from build123d import *

# Parameters (mm, degrees)
SKETCH008_W       = 45.6
SKETCH008_H       = 150
PAD004_DEPTH      = 42
PAD004_DEPTH_BACK = 10
SKETCH009_R       = 4
POCKET003_DEPTH   = 52.001
POCKET004_DEPTH   = 7
POCKET005_DEPTH   = 7
SKETCH011_R       = 4
POCKET007_DEPTH   = 45.601


with BuildPart() as part:
    # Sketch008 → Pad004 (new body, two sides)
    with BuildSketch(Plane(origin=(0, 0, 0), x_dir=(-1, 0, 0), z_dir=(0, 1, 0))) as pad004_sk:
        with Locations((214, 75)):
            Rectangle(SKETCH008_W, SKETCH008_H)
    extrude(amount=PAD004_DEPTH)
    extrude(pad004_sk.sketch, amount=-PAD004_DEPTH_BACK)

    # Sketch009 (on Face6 of Pad004) → Pocket003 (cut, through all)
    with BuildSketch(Plane(origin=(0, 42, 0), x_dir=(1, 0, 0), z_dir=(0, 1, 0))):
        with Locations((-211.172606, -26)):
            Circle(SKETCH009_R)
        with Locations((-211.172606, -124)):
            Circle(SKETCH009_R)
    extrude(amount=-POCKET003_DEPTH, mode=Mode.SUBTRACT)

    # Sketch010 (on Face4 of Pocket003) → Pocket004 (cut)
    with BuildSketch(Plane.XZ.offset(10)):
        Polygon((-207.672606, 117.937822), (-204.172606, 124), (-207.672606, 130.062178), (-214.672606, 130.062178), (-218.172606, 124), (-214.672606, 117.937822), align=None)
        Polygon((-207.672606, 19.937822), (-204.172606, 26), (-207.672606, 32.062178), (-214.672606, 32.062178), (-218.172606, 26), (-214.672606, 19.937822), align=None)
    extrude(amount=-POCKET004_DEPTH, mode=Mode.SUBTRACT)

    # Sketch010 (on Face4 of Pocket003) → Pocket005 (cut)
    with BuildSketch(Plane.XZ.offset(10)):
        Polygon((-207.672606, 117.937822), (-204.172606, 124), (-207.672606, 130.062178), (-214.672606, 130.062178), (-218.172606, 124), (-214.672606, 117.937822), align=None)
        Polygon((-207.672606, 19.937822), (-204.172606, 26), (-207.672606, 32.062178), (-214.672606, 32.062178), (-218.172606, 26), (-214.672606, 19.937822), align=None)
    extrude(amount=-POCKET005_DEPTH, mode=Mode.SUBTRACT)

    # Sketch011 → Pocket007 (cut, through all)
    with BuildSketch(Plane(origin=(-191.2, 0, 0), x_dir=(0, -1, 0), z_dir=(-1, 0, 0))):
        with Locations((-16, 135)):
            Circle(SKETCH011_R)
        with Locations((-16, 75)):
            Circle(SKETCH011_R)
        with Locations((-16, 15)):
            Circle(SKETCH011_R)
    extrude(amount=POCKET007_DEPTH, mode=Mode.SUBTRACT)


solid = part.part
The listing builds one solid part. Answer for the finished solid, in the listing's coordinates (mm). A direction names the side the tool comes from. Round coordinates to 2 decimals unless told otherwise and drop trailing zeros. Loops run counter-clockwise (first coordinate to the right, second up) from the corner with the lowest first, then second, coordinate; pieces in that order, holes last. Notation, with made-up numbers: M -10.5,-19.75 L -0.5,-19.75 A27 cw -0.5,19.25 Z; hole C 34,2.5 d4. An arc over 180 degrees is marked long. Write each question's results on one line, items separated by ' | '. Start each with the question number.
1) Find section B-B on y = -5. Write down the section's boundary in (x, z), plus the area to 3 significant figures.
2) Straight lines are drawn through the part: probe 1 along Y at (x, z) = (-215, 135); probe 2 along X at (y, z) = (20.5, 124); probe 3 along Z at (x, y) = (-222.5, 16). For each, find the intervals that lie inside material, in ascending order.
3) Which of the six approach directions +Z, -Z, +X, -X, +Y, -Y give full straight-line access (tool end or side, diameter ignored) to faces 1 (the flat face through (-216.447, -6.549, 121.011)), 2 (the cylindrical face through (-213.68, 18.95, 17.7))?
4) Find section A-A on z = 75. Write down the section's boundary in (x, y).
5) This flat-tipped pin is pushed along its axis until it touches: pin 1 (5 mm diameter, centred on x = -211.17, z = 26, fed in from -Y). Where does it stop, or does it pass through?
6) Find section C-C on x = -222. Write down the section's boundary in (y, z).
7) Find section D-D on y = 18. Write down the section's boundary in (x, z), plus the area to 3 significant figures.
8) Determine the mould class of faces 3 (the cylindrical face through (-213.681, 16.867, 71.095)), 4 (the flat face through (-236.8, 22, 74)), 5 (the flat face through (-211, -7, 19.938)) for opening direction X: pulls with the +X half, pulls with the -X half, needs draft (parallel to the pull), parting line crosses it, or undercut.
Final values:
1) outline: M -236.8,0 L -191.2,0 L -191.2,150 L -236.8,150 Z; hole M -218.17,26 L -214.67,19.94 L -207.67,19.94 L -204.17,26 L -207.67,32.06 L -214.67,32.06 Z; hole M -218.17,124 L -214.67,117.94 L -207.67,117.94 L -204.17,124 L -207.67,130.06 L -214.67,130.06 Z | area: 6,590 mm²
2) probe 1: -10 to 12, 20 to 42 | probe 2: -236.8 to -215.17, -207.17 to -191.2 | probe 3: 0 to 11, 19 to 71, 79 to 131, 139 to 150
3) face 1: -Y | face 2: +X, -X
4) outline: M -236.8,-10 L -191.2,-10 L -191.2,12 L -236.8,12 Z; M -236.8,20 L -191.2,20 L -191.2,42 L -236.8,42 Z
5) pin 1: through
6) outline: M -10,0 L 42,0 L 42,150 L -10,150 Z; hole C 16,15 d8; hole C 16,75 d8; hole C 16,135 d8
7) outline: M -236.8,0 L -191.2,0 L -191.2,11.54 L -236.8,11.54 Z; M -236.8,18.46 L -191.2,18.46 L -191.2,71.54 L -236.8,71.54 Z; M -236.8,78.46 L -191.2,78.46 L -191.2,131.54 L -236.8,131.54 Z; M -236.8,138.46 L -191.2,138.46 L -191.2,150 L -236.8,150 Z; hole C -211.17,26 d8; hole C -211.17,124 d8 | area: 5,790 mm²
8) face 3: needs draft | face 4: pulls with the -X half | face 5: undercut
